```python
from build123d import *

# Parameters (mm, degrees)
F1_DEPTH = 60
F2_R     = 3.5
F2_R_2   = 29
F3_DEPTH = 20
F4_T     = -2.5
F5_DEPTH = 40


with BuildPart() as f1:
    # F0 (on Front) → F1 (new body, symmetric)
    with BuildSketch(Plane.XZ):
        Polygon((-34.6706601963, 0), (65.0272384259, 0), (121.2443062928, 56.2170678669), (15.1782891148, 162.2830850448), (-90.8877280632, 56.2170678669), align=None)
    extrude(amount=F1_DEPTH, both=True)

    # F2 (on face) → F3 (cut)
    with BuildSketch(Plane(origin=(88.7306870798, 0, 88.7306870798), x_dir=(0.7071067812, 0, -0.7071067812), z_dir=(0.7071067812, 0, 0.7071067812))):
        with BuildLine():
            ThreePointArc((26.0637215376, 41.2), (25.4779351, 42.6142135624), (24.0637215376, 43.2))
            Line((24.0637215376, 43.2), (-80.4362784624, 43.2))
            ThreePointArc((-80.4362784624, 43.2), (-81.8504920248, 42.6142135624), (-82.4362784624, 41.2))
            Line((-82.4362784624, 41.2), (-82.4362784624, -41.2))
            ThreePointArc((-82.4362784624, -41.2), (-81.8504920248, -42.6142135624), (-80.4362784624, -43.2))
            Line((-80.4362784624, -43.2), (24.0637215376, -43.2))
            ThreePointArc((24.0637215376, -43.2), (25.4779351, -42.6142135624), (26.0637215376, -41.2))
            Line((26.0637215376, -41.2), (26.0637215376, 41.2))
        make_face()
        with Locations((-74.9362784624, -35.7)):
            Circle(F2_R, mode=Mode.SUBTRACT)
        with Locations((18.5637215376, -35.7)):
            Circle(F2_R, mode=Mode.SUBTRACT)
        with Locations((-74.9362784624, 35.7)):
            Circle(F2_R, mode=Mode.SUBTRACT)
        with Locations((-9.7362784624, 0)):
            Circle(F2_R_2, mode=Mode.SUBTRACT)
        with Locations((18.5637215376, 35.7)):
            Circle(F2_R, mode=Mode.SUBTRACT)
        with Locations((-9.7362784624, 0)):
            Circle(F2_R_2)
        with Locations((-74.9362784624, -35.7)):
            Circle(F2_R)
        with Locations((-74.9362784624, 35.7)):
            Circle(F2_R)
        with Locations((18.5637215376, 35.7)):
            Circle(F2_R)
        with Locations((18.5637215376, -35.7)):
            Circle(F2_R)
    extrude(amount=-F3_DEPTH, mode=Mode.SUBTRACT)

    # F4
    f4_openings = [f1.faces().sort_by_distance(p)[0] for p in [
        (15.178289, 0, 0),
    ]]
    offset(amount=F4_T, openings=f4_openings, kind=Kind.INTERSECTION)

    # F2 (on face) → F5 (cut)
    with BuildSketch(Plane(origin=(88.7306870798, 0, 88.7306870798), x_dir=(0.7071067812, 0, -0.7071067812), z_dir=(0.7071067812, 0, 0.7071067812))):
        with Locations((-9.7362784624, 0)):
            Circle(F2_R_2)
        with Locations((-74.9362784624, 35.7)):
            Circle(F2_R)
        with Locations((-74.9362784624, -35.7)):
            Circle(F2_R)
        with Locations((18.5637215376, -35.7)):
            Circle(F2_R)
        with Locations((18.5637215376, 35.7)):
            Circle(F2_R)
    extrude(amount=-F5_DEPTH, mode=Mode.SUBTRACT)


solid = f1.part
```
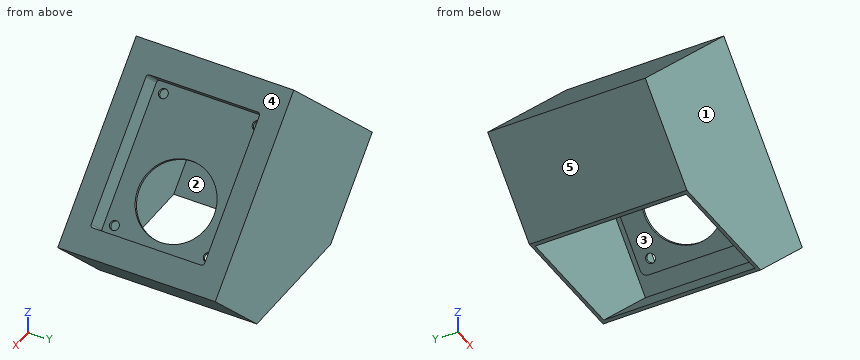
The model under review builds one solid part; all positions refer to its coordinate system, in mm. Face numbers are marked on the shaded views. A direction names the side the tool comes from. Round coordinates to 2 decimals unless told otherwise and drop trailing zeros. Order: outer loops, then holes, each group sorted by start corner. A loop starts at its lowest first (then second) coordinate and runs counter-clockwise, first axis right, second up. Notation, with made-up numbers: (7, 51) -> (22, 51) arc R14 ccw to (22, 67) -> close; hole circle Ø4 at (-29, -35.75). An arc over 180 degrees is marked (long way). One line per item, written item: value. Start each with the question number.
Q1. Take a section at B-B (x = -51.5). Write out the cut boundary in (y, z), and give its area (3 significant figures).
Q2. Take a section at C-C (y = 6). Write out the cut boundary in (x, z).
Q3. Take a section at A-A (y = -26). Write out the cut boundary in (x, z), and give its area (3 significant figures).
Q4. Wall thickness on line 1 (Y direction, x = 56.5, z = 116.5); line 2 (Y direction, x = 19, z = 19.5); line 3 (Y direction, x = 15.5, z = 132): over which ranges is each line inside the solid? List them lowest first.
Q5. Clearance check with flat-ended pins moving along their axes: pin 1 Ø12 at (x, y) = (-39.5, -35) entering from -Z; pin 2 Ø8 at (x, y) = (96, 39.5) entering from -Z; pin 3 Ø3 at (y, z) = (-23.5, 130.5) entering from -X; pin 4 Ø8 at (y, z) = (-41.5, 111) entering from -X. State where each tip first meets the part, or that it passes through.
Q6. Machinability: for the marked faces 1 and 2, which of the approach directions +Z, -Z, +X, -X, +Y, -Y give a long, thin tool a straight path to every point of the face, cutting with its end or side? Answer none if there is none.
Q7. Take a section at D-D (x = -11). Write out the cut boundary in (y, z).
Q8. Mouldability with a two-part tool opening along X and no side actions: class the marked faces 3, 4 and 5 as released by +X, released by -X, zero draft, split by the parting line, or undercut.
Reported:
1. outline: (-60, 16.83) -> (60, 16.83) -> (60, 95.6) -> (-60, 95.6) -> close; hole (-57.5, 20.36) -> (57.5, 20.36) -> (57.5, 92.07) -> (-57.5, 92.07) -> close
1. area: 1,210 mm2
2. outline: (-90.89, 56.22) -> (-34.67, 0) -> (-31.14, 0) -> (-87.35, 56.22) -> (15.18, 158.75) -> (26.9, 147.02) -> (12.76, 132.88) -> (45.87, 99.77) -> (47.64, 101.54) -> (16.3, 132.88) -> (30.44, 147.02) -> (15.18, 162.28) -> close; (61.49, 0) -> (65.03, 0) -> (121.24, 56.22) -> (107.16, 70.3) -> (93.02, 56.16) -> (87.77, 61.41) -> (86, 59.64) -> (93.02, 52.62) -> (107.16, 66.77) -> (117.71, 56.22) -> close
3. outline: (-90.89, 56.22) -> (-34.67, 0) -> (-31.14, 0) -> (-87.35, 56.22) -> (15.18, 158.75) -> (26.9, 147.02) -> (12.76, 132.88) -> (56.85, 88.79) -> (58.62, 90.56) -> (16.3, 132.88) -> (30.44, 147.02) -> (15.18, 162.28) -> close; (61.49, 0) -> (65.03, 0) -> (121.24, 56.22) -> (107.16, 70.3) -> (93.02, 56.16) -> (76.79, 72.39) -> (75.02, 70.62) -> (93.02, 52.62) -> (107.16, 66.77) -> (117.71, 56.22) -> close
3. area: 1,170 mm2
4. line 1: y = -60 to -57.5, -45.7 to -43.2, 43.2 to 45.7, 57.5 to 60
4. line 2: y = -60 to -57.5, 57.5 to 60
4. line 3: y = -60 to -57.5, -45.26 to 45.26, 57.5 to 60
5. pin 1: stops at z = 0
5. pin 2: stops at z = 26.97
5. pin 3: stops at x = -18.1
5. pin 4: stops at x = -40.1
6. face 1: +Z, -Z, +X, -X, -Y
6. face 2: none
7. outline: (-60, 0) -> (-57.5, 0) -> (-57.5, 132.57) -> (57.5, 132.57) -> (57.5, 0) -> (60, 0) -> (60, 136.1) -> (-60, 136.1) -> close
8. face 3: undercut
8. face 4: released by +X
8. face 5: released by -X
